For this review, take the finished solid that the model builds, in its own axes (mm). Face numbers are marked on the shaded views. A direction names the side the tool comes from. Give positions to 0.01 mm unless a question says otherwise; leave off trailing zeros. Order: outer loops, then holes, each group sorted by start corner. A loop starts at its lowest first (then second) coordinate and runs counter-clockwise, first axis right, second up. Notation, with made-up numbers: (-7, 21) - (43, 21) arc R14 cw to (43, 36) - close; hole circle Ø6 at (2.25, 11.5). An arc over 180 degrees is marked (long way). Answer as a JSON object with one key per item and string values. Group by question number.
from build123d import *

# Parameters (mm, degrees)
SKETCH_2_W               = 35
SKETCH_2_H               = 50
EXTRUDE_1_DEPTH          = 30
CUT_EXTRUDE_1_DEPTH      = 43.793106922
CUT_EXTRUDE_1_DEPTH_BACK = 43.793106922
SKETCH_3_R               = 7.5
FILLET_1_R               = 5
FILLET_2_R               = 5
SKETCH_4_R               = 2.75
CUT_EXTRUDE_2_DEPTH      = 20
SKETCH_5_W               = 30
SKETCH_5_H               = 15
EXTRUDE_2_DEPTH          = 10


with BuildPart() as part:
    # 草图2 → 凸台-拉伸1 (new body)
    with BuildSketch(Plane(origin=(0, 0, 0), x_dir=(0, 0, -1), z_dir=(1, 0, 0))):
        Rectangle(SKETCH_2_W, SKETCH_2_H)
    extrude(amount=EXTRUDE_1_DEPTH)

    # 草图3 → 切除-拉伸1 (cut, two sides: drawn at the far end of the back side and taken through both)
    with BuildSketch(Plane(origin=(30, 0, 0), x_dir=(0, 0, -1), z_dir=(1, 0, 0)).offset(-CUT_EXTRUDE_1_DEPTH_BACK)):
        with Locations((0, -5)):
            Circle(SKETCH_3_R)
    extrude(amount=CUT_EXTRUDE_1_DEPTH + CUT_EXTRUDE_1_DEPTH_BACK, mode=Mode.SUBTRACT)

    # 圆角1
    fillet_1_edges = [part.edges().sort_by_distance(p)[0] for p in [
        (15, -25, -17.5),
    ]]
    fillet(fillet_1_edges, radius=FILLET_1_R)

    # 圆角2
    fillet_2_edges = [part.edges().sort_by_distance(p)[0] for p in [
        (15, -25, 17.5),
    ]]
    fillet(fillet_2_edges, radius=FILLET_2_R)

    # 草图4 → 切除-拉伸2 (cut)
    with BuildSketch(Plane.ZY):
        with Locations((11.313708499, 6.313708499)):
            Circle(SKETCH_4_R)
        with Locations((-11.313708499, 6.313708499)):
            Circle(SKETCH_4_R)
        with Locations((-11.313708499, -16.313708499)):
            Circle(SKETCH_4_R)
        with Locations((11.313708499, -16.313708499)):
            Circle(SKETCH_4_R)
    extrude(amount=-CUT_EXTRUDE_2_DEPTH, mode=Mode.SUBTRACT)

    # 草图5 → 凸台-拉伸2 (add)
    with BuildSketch(Plane(origin=(0, 25, 0), x_dir=(1, 0, 0), z_dir=(0, 1, 0))):
        with Locations((15, -25)):
            Rectangle(SKETCH_5_W, SKETCH_5_H)
    extrude(amount=-EXTRUDE_2_DEPTH)


solid = part.part
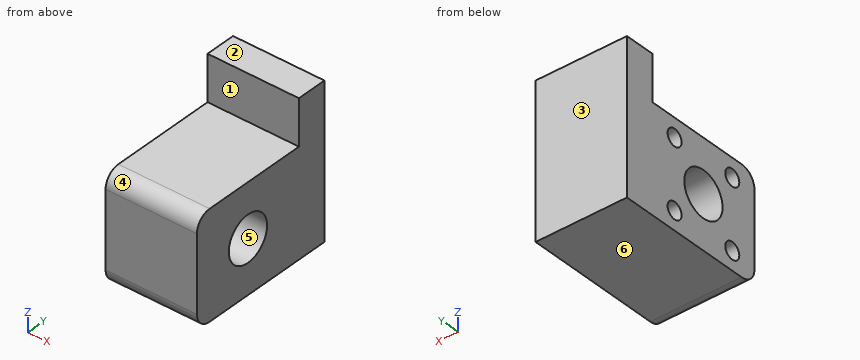
1) For the marked faces 1 and 2, list the 3-axis set-ups (+Z, -Z, +X, -X, +Y, -Y) from which the entire face can be reached by the end or side of a thin tool; tool diameter is ignored.
2) Consider section C-C (x = 24.75). Give the boundary of the cut face in (y, z).
3) Consider section A-A (z = 0). Give the boundary of the cut face in (x, y).
4) Mouldability with a two-part tool opening along Z and no side actions: class the marked faces 3, 4, 5 and 6 as released by +Z, released by -Z, zero draft, split by the parting line, or undercut.
5) For pin 1 (3 mm diameter, centred on y = 6, z = 11.5, fed in from -X); pin 2 (6 mm diameter, centred on y = -15, z = 11.5, fed in from -X); pin 3 (4.5 mm diameter, centred on x = 16, z = 23, fed in from -Y); pin 4 (1 mm diameter, centred on x = 8.5, y = 4.5, fed in from +Z), all flat-tipped, find the tip position at first contact; note any pin that passes through.
6) Consider section D-D (y = 5). Give the boundary of the cut face in (x, z).
7) Consider section B-B (y = -5). Give the boundary of the cut face in (x, z).
8) For line 1 (Y direction, x = 15.5, z = 9.5); line 2 (Z direction, x = 11, y = 5); line 3 (Z direction, x = 4.25, y = 0.5), list the stretches that pass through material, from the lowest coordinate up.
Result set:
{
 "1": {"face 1": "+Z, +X, -X, -Y", "face 2": "+Z, +X, -X, +Y, -Y"},
 "2": {"outline": "(-25, -12.5) arc R5 ccw to (-20, -17.5) - (25, -17.5) - (25, 32.5) - (15, 32.5) - (15, 17.5) - (-20, 17.5) arc R5 ccw to (-25, 12.5) - close; hole circle Ø15 at (-5, 0)"},
 "3": {"outline": "(0, -25) - (30, -25) - (30, -12.5) - (0, -12.5) - close; (0, 2.5) - (30, 2.5) - (30, 25) - (0, 25) - close"},
 "4": {"face 3": "zero draft", "face 4": "released by +Z", "face 5": "undercut", "face 6": "released by -Z"},
 "5": {"pin 1": "stops at x = 20", "pin 2": "stops at x = 0", "pin 3": "stops at y = 15", "pin 4": "stops at z = 17.5"},
 "6": {"outline": "(0, -17.5) - (30, -17.5) - (30, 17.5) - (0, 17.5) - (0, 13.73) - (20, 13.73) - (20, 8.9) - (0, 8.9) - (0, -8.9) - (20, -8.9) - (20, -13.73) - (0, -13.73) - close"},
 "7": {"outline": "(0, -17.5) - (30, -17.5) - (30, -7.5) - (0, -7.5) - close; (0, 7.5) - (30, 7.5) - (30, 17.5) - (0, 17.5) - close"},
 "8": {"line 1": "y = -25 to -18.38, -14.25 to 4.25, 8.38 to 25", "line 2": "z = -17.5 to -13.73, -8.9 to 8.9, 13.73 to 17.5", "line 3": "z = -17.5 to -5.1, 5.1 to 17.5"}
}
